Autodesk Inventor part; units mm, degrees
ref_plane "YZ Plane" through (0, 0, 0) normal (1, 0, 0) x (0, 1, 0)
ref_plane "XZ Plane" through (0, 0, 0) normal (0, 1, 0) x (-1, 0, 0)
ref_plane "XY Plane" through (0, 0, 0) normal (0, 0, 1) x (1, 0, 0)
sketch "Esquisse1" plane through (0, 0, 0) normal (0, 1, 0) x (-1, 0, 0)
  line L0 (-61.8861, -256.597) -> (-116.8861, -256.597)
  line L1 (-116.8861, -256.597) -> (-116.8861, -296.597)
  line L2 (-116.8861, -296.597) -> (-61.8861, -296.597)
  arc A0 (-61.8861, -296.597) -> (-61.8861, -256.597) centre (-61.8861, -276.597) ccw
  dimension "d1" = 40
  dimension "d2" = 55
  dimension "d3" = 55
extrude "Extrusion1" add sketch "Esquisse1" along normal blind 10
sketch "Esquisse3" plane through (0, 0, 0) normal (0, -1, 0) x (1, 0, 0)
  line L0 (89.3861, -269.097) -> (104.3861, -269.097)
  line L1 (104.3861, -269.097) -> (104.3861, -284.097)
  line L2 (104.3861, -284.097) -> (89.3861, -284.097)
  line L3 (89.3861, -284.097) -> (89.3861, -269.097)
  line L4 (116.8861, -296.597) -> (61.8861, -296.597)
  line L5 (116.8861, -256.597) -> (116.8861, -296.597)
  point P0 (0, 0)
  dimension "d19" = 15
  dimension "d20" = 15
  dimension "d21" = 12.5
  dimension "d22" = 12.5
extrude "Extrusion3" add sketch "Esquisse3" along normal blind 15
chamfer "Chanfrein2" distance 4 angle 45 4 edges at (89.3861, -7.5, -284.097) (104.3861, -7.5, -284.097) (89.3861, -7.5, -269.097) (104.3861, -7.5, -269.097)
sketch "Esquisse4" plane through (0, 10, 0) normal (0, 1, 0) x (1, 0, 0)
  line L0 (116.8861, 296.597) -> (61.8861, 296.597)
  arc A0 (61.8861, 296.597) -> (61.8861, 256.597) centre (61.8861, 276.597) ccw
  circle A1 centre (61.8861, 276.597) radius 19
  point P0 (0, 0)
  dimension "d28" = 1
extrude "Extrusion4" add sketch "Esquisse4" along normal blind 73
chamfer "Chanfrein3" distance 10 angle 45 2 edges at (116.8861, 5, -256.597) (116.8861, 5, -296.597)
sketch "Esquisse5" plane through (0, 10, 0) normal (0, 1, 0) x (1, 0, 0)
  line L0 (61.8861, 256.597) -> (106.8861, 256.597)
  line L1 (106.8861, 296.597) -> (61.8861, 296.597)
  arc A0 (97.6044, 288.5312) -> (97.6044, 264.6628) centre (93.8861, 276.597) ccw
  circle A1 centre (61.8861, 276.597) radius 19
  line L2 (116.8861, 266.597) -> (116.8861, 286.597)
  line L3 (116.8861, 267.597) -> (116.8861, 285.597)
  line L4 (116.8861, 267.597) -> (93.8861, 264.097)
  line L5 (116.8861, 285.597) -> (93.8861, 289.097)
  point P0 (0, 0)
  dimension "d34" = 25
  dimension "d35" = 32
  dimension "d36" = 1
  dimension "d37" = 1
extrude "Extrusion5" add sketch "Esquisse5" along normal blind 110 contours L5 L2 L4 A0
sketch "Esquisse6" plane through (0, 120, 0) normal (0, 1, 0) x (1, 0, 0)
  line L0 (116.8861, 267.597) -> (93.8861, 264.097)
  arc A0 (93.8861, 289.097) -> (93.8861, 264.097) centre (93.8861, 276.597) ccw
  line L1 (93.8861, 264.097) -> (93.8861, 264.097)
  circle A1 centre (93.8861, 276.597) radius 10
  point P0 (0, 0)
  dimension "d40" = 20
extrude "Extrusion6" add sketch "Esquisse6" along normal blind 22
ref_plane "Plan de construction1" through (61.8861, 0, -276.597) normal (0, 0, -1) x (-1, 0, 0)
sketch "Esquisse7" plane through (61.8861, 0, -276.597) normal (0, 0, -1) x (-1, 0, 0)
  point P0 (61.8861, 0)
sketch "Esquisse8" plane through (0, 0, 0) normal (0, -1, 0) x (1, 0, 0)
  point P0 (0, 0)
sketch "Esquisse9" plane through (0, 0, 0) normal (0, -1, 0) x (1, 0, 0)
  arc A0 (61.8861, -256.597) -> (61.8861, -296.597) centre (61.8861, -276.597) ccw
  line L0 (61.8861, -256.597) -> (106.8861, -256.597)
  line L1 (106.8861, -256.597) -> (116.8861, -266.597)
  line L2 (116.8861, -266.597) -> (116.8861, -286.597)
  line L3 (116.8861, -286.597) -> (106.8861, -296.597)
  line L4 (106.8861, -296.597) -> (61.8861, -296.597)
  line L5 (61.8861, -256.597) -> (106.8861, -256.597)
  line L6 (61.8861, -255.597) -> (106.8861, -255.597)
  line L7 (106.8861, -255.597) -> (117.5932, -265.8899)
  line L8 (117.5932, -265.8899) -> (117.5932, -287.3041)
  line L9 (117.5932, -287.3041) -> (106.8861, -297.597)
  line L10 (106.8861, -297.597) -> (61.8861, -297.597)
  arc A1 (61.8861, -255.597) -> (61.8861, -297.597) centre (61.8861, -276.597) ccw
  line L11 (108.8997, -250.597) -> (61.8861, -250.597)
  arc A2 (61.8861, -250.597) -> (61.8861, -302.597) centre (61.8861, -276.597) ccw
  line L12 (61.8861, -302.597) -> (108.8997, -302.597)
  line L13 (108.8997, -302.597) -> (122.5932, -289.4332)
  line L14 (122.5932, -289.4332) -> (122.5932, -263.7609)
  line L15 (122.5932, -263.7609) -> (108.8997, -250.597)
  point P0 (0, 0)
  dimension "d51" = 1
  dimension "d52" = 1
  dimension "d53" = 1
  dimension "d54" = 5
extrude "Extrusion7" add sketch "Esquisse9" against normal blind 85 contours L15 L14 L13 L12 A2 L11
sketch "Esquisse10" plane through (0, 0, 0) normal (0, -1, 0) x (1, 0, 0)
  line L0 (89.3861, -273.097) -> (89.3861, -280.097)
  line L1 (104.3861, -280.097) -> (104.3861, -273.097)
  line L2 (61.8861, -302.597) -> (108.8997, -302.597)
  line L3 (89.3861, -250.597) -> (89.3861, -263.7609)
  line L4 (89.3861, -302.597) -> (79.3861, -302.597)
  line L5 (79.3861, -302.597) -> (79.3861, -250.597)
  line L6 (122.5932, -263.7609) -> (89.3861, -263.7609)
  line L7 (89.3861, -268.7609) -> (122.5932, -268.7609)
  line L8 (122.5932, -289.4332) -> (89.3861, -289.4332)
  line L9 (89.3861, -284.4332) -> (122.5932, -284.4332)
  line L10 (89.3861, -289.4332) -> (89.3861, -302.597)
  line L11 (89.3861, -268.7609) -> (89.3861, -284.4332)
  line L12 (79.3861, -250.597) -> (89.3861, -250.597)
  line L13 (108.8997, -250.597) -> (61.8861, -250.597)
  line L14 (122.5932, -263.7609) -> (122.5932, -268.7609)
  line L15 (122.5932, -284.4332) -> (122.5932, -289.4332)
  point P0 (0, 0)
  dimension "d57" = 10
  dimension "d58" = 5
  dimension "d59" = 5
extrude "Extrusion8" add sketch "Esquisse10" along normal blind 15
sketch "Esquisse11" plane through (0, 85, 0) normal (0, 1, 0) x (1, 0, 0)
  line L0 (116.8861, 286.597) -> (114.0499, 289.4332)
  line L1 (116.8861, 286.597) -> (116.8861, 266.597)
  line L2 (61.8861, 256.597) -> (106.8861, 256.597)
  line L3 (106.8861, 256.597) -> (61.8861, 256.597)
  line L4 (114.0499, 289.4332) -> (106.8861, 296.597)
  line L5 (106.8861, 296.597) -> (61.8861, 296.597)
  line L6 (106.8861, 296.597) -> (61.8861, 296.597)
  line L7 (61.8861, 296.597) -> (106.8861, 296.597)
  line L8 (106.8861, 296.597) -> (116.8861, 286.597)
  arc A0 (61.8861, 296.597) -> (61.8861, 256.597) centre (61.8861, 276.597) ccw
  line L9 (114.0499, 263.7609) -> (116.8861, 266.597)
  line L10 (116.8861, 266.597) -> (106.8861, 256.597)
  point P0 (0, 0)
extrude "Extrusion9" cut sketch "Esquisse11" against normal blind 85 and the other way blind 42.5
sketch "Esquisse12" plane through (93.8861, 127.5, -276.597) normal (0, -1, 0) x (1, 0, 0)
  point P0 (-93.8861, 276.597)
sketch "Esquisse13" plane through (93.8861, 142, -276.597) normal (0, 1, 0) x (1, 0, 0)
  circle A0 centre (0, 0) radius 10.5
  point P0 (-93.8861, -276.597)
  dimension "d66" = 21
extrude "Extrusion10" cut sketch "Esquisse13" against normal blind 85
sketch "Esquisse14" plane through (0, -15, 0) normal (0, -1, 0) x (1, 0, 0)
  line L0 (89.3861, -284.4332) -> (89.3861, -280.097)
  line L1 (89.3861, -268.7609) -> (122.5932, -268.7609)
  line L2 (89.3861, -284.4332) -> (113.204, -284.4332)
  line L3 (113.204, -284.4332) -> (113.204, -268.7609)
  line L4 (113.204, -268.7609) -> (89.3861, -268.7609)
  line L5 (89.3861, -268.7609) -> (89.3861, -284.4332)
  point P0 (0, 0)
extrude "Extrusion11" cut sketch "Esquisse14" against normal blind 85
sketch "Esquisse17" plane through (61.8861, 85, -250.597) normal (0, 0, 1) x (1, 0, 0)
  line L0 (0, 0) -> (10, 0)
  line L1 (10, 0) -> (10, -8)
  line L2 (10, -8) -> (0, -8)
  line L3 (0, -8) -> (0, 0)
  line L4 (10, 0) -> (20, 0)
  line L5 (0, 0) -> (47.0135, 0)
  line L6 (20, 0) -> (30, 0)
  line L7 (30, 0) -> (30, -8)
  line L8 (30, -8) -> (20, -8)
  line L9 (20, -8) -> (20, 0)
  point P0 (-61.8861, -85)
  dimension "d79" = 10
  dimension "d80" = 8
  dimension "d81" = 10
  dimension "d82" = 10
extrude "Extrusion13" add sketch "Esquisse17" along normal blind 30
sketch "Esquisse18" plane through (81.8861, 77, -250.597) normal (0, -1, 0) x (1, 0, 0)
  line L0 (10, 30) -> (0, 30)
  point P0 (-81.8861, 250.597)
  point P1 (5, 22)
  point P2 (5, 10)
ref_plane "Plan de construction2" through (76.8861, 77, -250.597) normal (-1, 0, 0) x (0, 0, 1)
hole "Perçage1" at (86.8861, 77, -240.597) at (86.8861, 77, -228.597) direction (0, 1, 0) diameter 4 end through all
mirror "Symétrie1" about plane through (76.8861, 77, -250.597) normal (-1, 0, 0) of "Perçage1"
mirror "Symétrie2" about plane through (61.8861, 0, -276.597) normal (0, 0, -1) of "Extrusion13", "Perçage1", "Symétrie1"
sketch "Esquisse19" plane through (0, 0, 0) normal (0, -1, 0) x (1, 0, 0)
  line L0 (61.8861, -302.597) -> (79.3861, -302.597)
  line L1 (61.8861, -302.597) -> (131.8861, -302.597)
  line L2 (131.8861, -302.597) -> (131.8861, -247.7831)
  line L3 (131.8861, -247.7831) -> (61.8861, -247.7831)
  line L4 (61.8861, -247.7831) -> (61.8861, -302.597)
  point P0 (0, 0)
  point P1 (61.8861, -250.597)
  dimension "d95" = 70
extrude "Extrusion14" cut sketch "Esquisse19" along normal blind 15
sketch "Esquisse20" plane through (0, 0, 0) normal (0, -1, 0) x (1, 0, 0)
  line L0 (61.8861, -250.597) -> (61.8861, -220.597)
  arc A0 (61.8861, -255.597) -> (61.8861, -297.597) centre (61.8861, -276.597) ccw
  line L1 (61.8861, -250.597) -> (61.8861, -255.597)
  line L2 (61.8861, -297.597) -> (61.8861, -303.2676)
  line L3 (61.8861, -302.597) -> (71.8861, -302.597)
  arc A1 (61.8861, -250.597) -> (61.8861, -302.597) centre (61.8861, -276.597) ccw
  arc A2 (61.8861, -255.597) -> (61.8861, -297.597) centre (61.8861, -276.597) ccw
  point P0 (0, 0)
extrude "Extrusion15" cut sketch "Esquisse20" against normal blind 20
equation "\"d93\" = Epaisseur"
equation "\"RayonPli\" = Epaisseur"
equation "\"LargeurGrugeage\" = Epaisseur"
equation "\"ProfondeurGrugeage\" = 0.5 * Epaisseur"
equation "\"TailleGrugeage\" = 4 * Epaisseur"
equation "\"RestesMinimum\" = 2 * Epaisseur"
equation "\"Rayondetransition\" = RayonPli"
equation "\"TailleRayonJacobi\" = Epaisseur"
equation "\"TailleJeu\" = Epaisseur"
properties part number "actionneur linéaire"
Can you work these out from the model? Positions are in its coordinate system, mm. A direction names the side the tool comes from. Coordinates: 2 decimals unless noted, no trailing zeros. Write each loop counter-clockwise with the first axis right and the second up, starting at its lowest first coordinate (ties: lowest second). Pieces come first, ordered by that corner, then holes. Notation, with made-up numbers: (14.5, 20.5) -> (41.5, 20.5) arc R29 ccw to (41.5, 44.5) -> close; hole circle Ø7 at (-16, -35.5). An arc over 180 degrees is marked (long way). Write each question's results on one line, items separated by ' | '. Start each with the question number.
Item 1: If we section it at A-A, the plane x = 103: Write out the boundary of the cut face in (y, z).
Item 2: If we section it at B-B, the plane z = -304: Write out the boundary of the cut face in (x, y), and give its area (3 significant figures).
Item 3: If we section it at C-C, the plane y = 27: Write out the boundary of the cut face in (x, z).
Item 4: Thinking about a two-plate mould opening in Z: for faces 1 (the flat face through (117.593, 42, -276)), 2 (the flat face through (61.886, 10, -300)), 3 (the flat face through (87, 81, -220.597)), which applies, released by +Z, released by -Z, zero draft, split by the parting line, or undercut?
Item 5: I'm going to push flat-ended pins straight in: P1, Ø12, axis at y = 29.5, z = -281, coming from the -X side; P2, Ø1, axis at x = 93, y = 27.5, coming from the +Z side; P3, Ø9, axis at y = 79.5, z = -319.5, coming from the -X side; P4, Ø3.5, axis at x = 66.89, z = -312.6, coming from the +Y side. Where does each tip first touch, or does it pass through?
Item 6: Please list where these lines run through material, in increasing order: probe 1 along Z at (x, y) = (68.5, 49.5); probe 2 along X at (y, z) = (79, -282.5); probe 3 along Z at (x, y) = (60, 24.5).
Item 7: On a 3-axis mill with a long thin cutter (end or side, diameter ignored), from which of +Z, -Z, +X, -X, +Y, -Y can I reach the whole of each face in a straight line? I mean faces 4 (the flat face through (71.886, 81, -317)), 5 (the flat face through (84, 42, -255.597)), 6 (the flat face through (87, 77, -317)), 7 (the flat face through (91.886, 81, -236)), 8 (the flat face through (71.886, 81, -236)). Say none if no direction works.
Answer block:
1) outline: (0, -302.6) -> (85, -302.6) -> (85, -297.6) -> (0, -297.6) -> close; (0, -255.6) -> (85, -255.6) -> (85, -250.6) -> (0, -250.6) -> close
2) outline: (61.89, 77) -> (71.89, 77) -> (71.89, 85) -> (61.89, 85) -> close; (81.89, 77) -> (91.89, 77) -> (91.89, 85) -> (81.89, 85) -> close | area: 160 mm²
3) outline: (61.89, -302.6) -> (108.9, -302.6) -> (122.59, -289.43) -> (122.59, -263.76) -> (108.9, -250.6) -> (61.89, -250.6) arc R26 ccw to start; hole (61.89, -297.6) -> (106.89, -297.6) -> (117.59, -287.3) -> (117.59, -265.89) -> (106.89, -255.6) -> (61.89, -255.6) arc R21 ccw to start
4) face 1: undercut | face 2: zero draft | face 3: released by +Z
5) P1: x = 35.89 | P2: z = -250.6 | P3: x = 61.89 | P4: through
6) probe 1: -302.6 to -297.6, -255.6 to -250.6 | probe 2: 36.57 to 41.73, 117.59 to 122.59 | probe 3: -302.53 to -297.51, -255.68 to -250.67
7) face 4: -Z, +Y, -Y | face 5: +Y, -Y | face 6: -Z, +X, -X, -Y | face 7: +Z, +X, +Y, -Y | face 8: +Z, +Y, -Y
